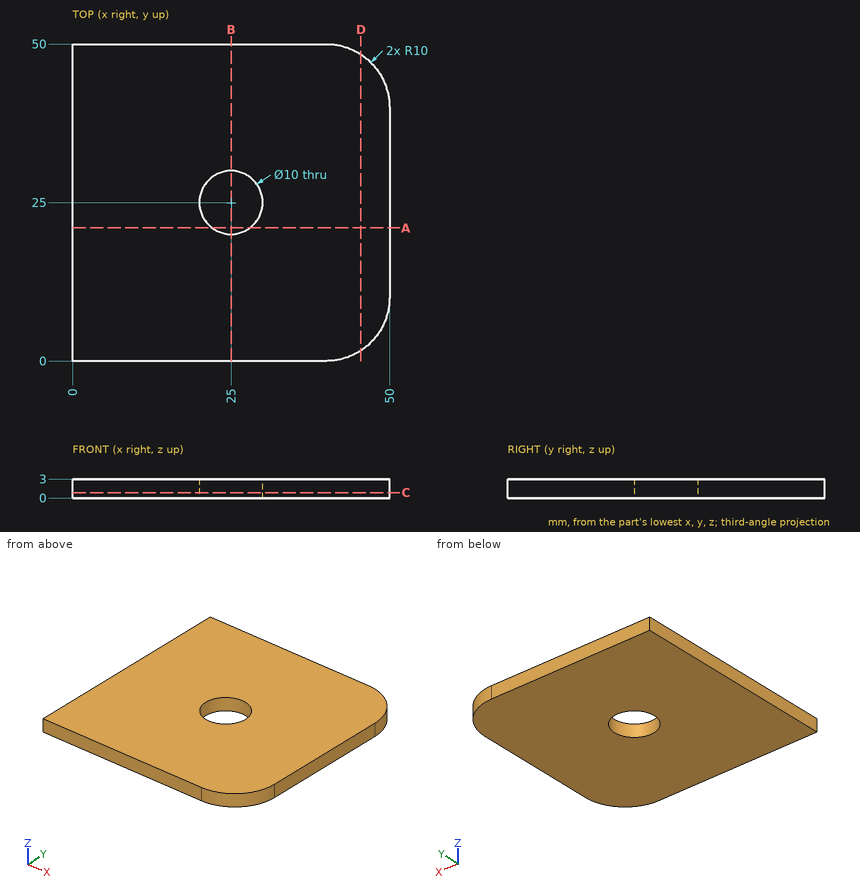
Verification items for this drawing (mm, ordinates from the low corner). Give positions to 0.01 mm unless a question says otherwise; leave off trailing zeros. Loops run counter-clockwise (first coordinate to the right, second up) from the corner with the lowest first, then second, coordinate; pieces in that order, holes last. Notation, with made-up numbers: M 65,-34 L 98,-34 A18 cw 98,-9 Z; hole C 18,50.5 d8. An arc over 180 degrees is marked long. Write item = value, one per line. Start each with the question number.
1. Thickness scan on probe 1 along Y at (x, z) = (25, 0.65); probe 2 along X at (y, z) = (26, 2.85); probe 3 along X at (y, z) = (21.5, 1.95). Record the ranges inside material, lowest first.
2. Section check A-A, the plane y = 21. Enter the section's corners in (x, z), plus the area to 3 significant figures.
3. Section check D-D, the plane x = 45.5. Enter the section's corners in (y, z), plus the area to 3 significant figures.
4. Section check B-B, the plane x = 25. Enter the section's corners in (y, z).
5. Go/stop test with a flat-tipped pin: P1, Ø6, axis at x = 25, y = 25, coming from the +Z side. Record where the tip stops, or that it passes through.
6. Section check C-C, the plane z = 0.85. Enter the section's corners in (x, y).
Values follow:
q1.probe_1 = 0 to 20, 30 to 50
q1.probe_2 = 0 to 20.1, 29.9 to 50
q1.probe_3 = 0 to 21.43, 28.57 to 50
q2.outline = M 0,0 L 22,0 L 22,3 L 0,3 Z; M 28,0 L 50,0 L 50,3 L 28,3 Z
q2.area = 132 mm^2
q3.outline = M 1.65,0 L 48.35,0 L 48.35,3 L 1.65,3 Z
q3.area = 140 mm^2
q4.outline = M 0,0 L 20,0 L 20,3 L 0,3 Z; M 30,0 L 50,0 L 50,3 L 30,3 Z
q5.P1 = through
q6.outline = M 0,0 L 40,0 A10 ccw 50,10 L 50,40 A10 ccw 40,50 L 0,50 Z; hole C 25,25 d10
